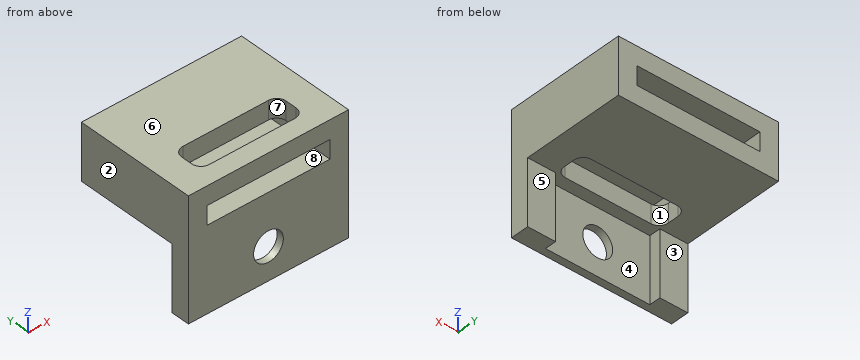
from build123d import *

# Parameters (mm, degrees)
SKETCH1_W           = 17.2
SKETCH1_H           = 6
SKETCH1_W_2         = 13.2
SKETCH1_H_2         = 2
BOSS_EXTRUDE1_DEPTH = 13
CUT_EXTRUDE1_DEPTH  = 13
SKETCH4_W           = 17.2
SKETCH4_H           = 1.968955047
BOSS_EXTRUDE2_DEPTH = 7
SKETCH5_R           = 1.6
CUT_EXTRUDE2_DEPTH  = 4
SKETCH6_W           = 11.206506984
SKETCH6_H           = 2.48590404
CUT_EXTRUDE3_DEPTH  = 7


with BuildPart() as part:
    # Sketch1 → Boss-Extrude1 (new body)
    with BuildSketch(Plane(origin=(0, 0, 0), x_dir=(1, 0, 0), z_dir=(0, 1, 0))):
        with Locations((6.6, 1)):
            Rectangle(SKETCH1_W, SKETCH1_H)
        with Locations((6.6, 1)):
            Rectangle(SKETCH1_W_2, SKETCH1_H_2, mode=Mode.SUBTRACT)
    extrude(amount=BOSS_EXTRUDE1_DEPTH)

    # Sketch2 → Cut-Extrude1 (cut)
    with BuildSketch(Plane.XY.offset(2)):
        with BuildLine():
            Line((2, 5.2), (11.2, 5.2))
            ThreePointArc((11.2, 5.2), (11.907106781, 4.907106781), (12.2, 4.2))
            Line((12.2, 4.2), (12.2, 3))
            ThreePointArc((12.2, 3), (11.907106781, 2.292893219), (11.2, 2))
            Line((11.2, 2), (2, 2))
            ThreePointArc((2, 2), (1.292893219, 2.292893219), (1, 3))
            Line((1, 3), (1, 4.2))
            ThreePointArc((1, 4.2), (1.292893219, 4.907106781), (2, 5.2))
        make_face()
    extrude(amount=-CUT_EXTRUDE1_DEPTH, mode=Mode.SUBTRACT)

    # Sketch4 → Boss-Extrude2 (add)
    with BuildSketch(Plane(origin=(0, 0, -4), x_dir=(-1, 0, 0), z_dir=(0, 0, -1))):
        with Locations((-6.6, 0.984477524)):
            Rectangle(SKETCH4_W, SKETCH4_H)
    extrude(amount=BOSS_EXTRUDE2_DEPTH)

    # Sketch5 → Cut-Extrude2 (cut)
    with BuildSketch(Plane(origin=(0, 1.968955047, 0), x_dir=(1, 0, 0), z_dir=(0, 1, 0))):
        with Locations((6.6, 7.5)):
            Circle(SKETCH5_R)
    extrude(amount=-CUT_EXTRUDE2_DEPTH, mode=Mode.SUBTRACT)

    # Sketch6 → Cut-Extrude3 (cut)
    with BuildSketch(Plane(origin=(0, 0, -11), x_dir=(-1, 0, 0), z_dir=(0, 0, -1))):
        with Locations((-6.603253492, 1.995400835)):
            Rectangle(SKETCH6_W, SKETCH6_H)
    extrude(amount=-CUT_EXTRUDE3_DEPTH, mode=Mode.SUBTRACT)


solid = part.part
Build history of the part. All positions in model axes, mm. Face numbers are marked on the shaded views. A direction names the side the tool comes from. Give positions to 0.01 mm unless a question says otherwise; leave off trailing zeros. Order: outer loops, then holes, each group sorted by start corner. A loop starts at its lowest first (then second) coordinate and runs counter-clockwise, first axis right, second up. Notation, with made-up numbers: M 46.5,-2 L 58.5,-2 A25 ccw 58.5,27 Z; hole C 40,55 d8. An arc over 180 degrees is marked long. Use one line per item in the form item = value.
Q1. Pull direction X, two halves, no side cores. Call the marked faces 1, 2 and 3: released by +X, released by -X, zero draft, split by the parting line, or undercut.
Conclusion:
face_1 = undercut
face_2 = released by -X
face_3 = zero draft
Q2. Slice it at D-D, the plane x = 6.6. Write the cut outline in (y, z).
Conclusion:
outline = M 0,-11 L 0.75,-11 L 0.75,-9.1 L 0,-9.1 Z; M 0,-5.9 L 0.75,-5.9 L 0.75,-4 L 2,-4 L 2,-2 L 0,-2 Z; M 0,0 L 2,0 L 2,2 L 0,2 Z; M 5.2,-4 L 13,-4 L 13,-2 L 5.2,-2 Z; M 5.2,0 L 13,0 L 13,2 L 5.2,2 Z
Q3. Wall check: probe 1 along Z at (x, y) = (6.6, 0.45); probe 2 along X at (y, z) = (3, 0.5); probe 3 along Y at (x, z) = (5.25, 1). Give the ranges that are in metal, low to high.
Conclusion:
probe_1 = -11 to -9.1, -5.9 to -2, 0 to 2
probe_2 = -2 to 1, 12.2 to 15.2
probe_3 = 0 to 2, 5.2 to 13
Q4. Pin check, flat tips, straight feed: P1, Ø1.5, axis at y = 5.5, z = -6.5, coming from the -X side; P2, Ø2, axis at x = 12.5, y = 4.5, coming from the -Z side; P3, Ø3.5, axis at x = 9, z = -7, coming from the +Y side; P4, Ø0.9, axis at x = -1, z = -7, coming from the +Y side. Stop position of each tip, or through.
Conclusion:
P1 = through
P2 = -4
P3 = 0.75
P4 = 1.97
Q5. Slice it at B-B, the plane y = 10. Write the cut outline in (x, z), and give its area (3 significant figures).
Conclusion:
outline = M -2,-4 L 15.2,-4 L 15.2,2 L -2,2 Z; hole M 0,-2 L 13.2,-2 L 13.2,0 L 0,0 Z
area = 76.8 mm2
Q6. Which spindle directions (+Z, -Z, +X, -X, +Y, -Y) get a long thin tool onto all of the face, cutting with end or side? Do the marked faces 4, 5, 6, 7 and 8. Say none if no direction does.
Conclusion:
face_4 = -Z, +Y
face_5 = -Z, +X, -X, +Y
face_6 = +Z, +X, -X, +Y, -Y
face_7 = +Z, -Z
face_8 = +Y, -Y
Q7. Slice it at C-C, the plane z = -7.5. Write the cut outline in (x, y).
Conclusion:
outline = M -2,0 L 5,0 L 5,0.75 L 1,0.75 L 1,1.97 L -2,1.97 Z; M 8.2,0 L 15.2,0 L 15.2,1.97 L 12.21,1.97 L 12.21,0.75 L 8.2,0.75 Z
Q8. Slice it at A-A, the plane x = 4.25. Write the cut outline in (y, z), and give its area (3 significant figures).
Conclusion:
outline = M 0,-11 L 0.75,-11 L 0.75,-4 L 2,-4 L 2,-2 L 0,-2 Z; M 0,0 L 2,0 L 2,2 L 0,2 Z; M 5.2,-4 L 13,-4 L 13,-2 L 5.2,-2 Z; M 5.2,0 L 13,0 L 13,2 L 5.2,2 Z
area = 44.5 mm2
